Source: three-view drawing plus pictorial views. Frame: mm from the lowest corner of the part. Round coordinates to 2 decimals unless told otherwise and drop trailing zeros. Order: outer loops, then holes, each group sorted by start corner. A loop starts at its lowest first (then second) coordinate and runs counter-clockwise, first axis right, second up. Notation, with made-up numbers: (82.25, -31.5) -> (117.25, -31.5) arc R13 ccw to (117.25, -7.5) -> close; hole circle Ø6 at (8, -32). An arc over 180 degrees is marked (long way). Answer as CSV lines item,"result". Start each with the question number.
1) Line query: L1, parallel to Y at x = 105, z = 2.1; L2, parallel to X at y = 45, z = 2.2; L3, parallel to Y at x = 45, z = 1.8. Output: solid intervals per line, ascending.
2) Section query A-A, the plane y = 49.5. Output: boundary loops of the cut face in (x, z), and give its area (3 significant figures).
3) First-contact query: P1, Ø4, axis at x = 120, y = 60, coming from the +Z side. Flat tip, straight axial feed; report the tip coordinate or a pass-through.
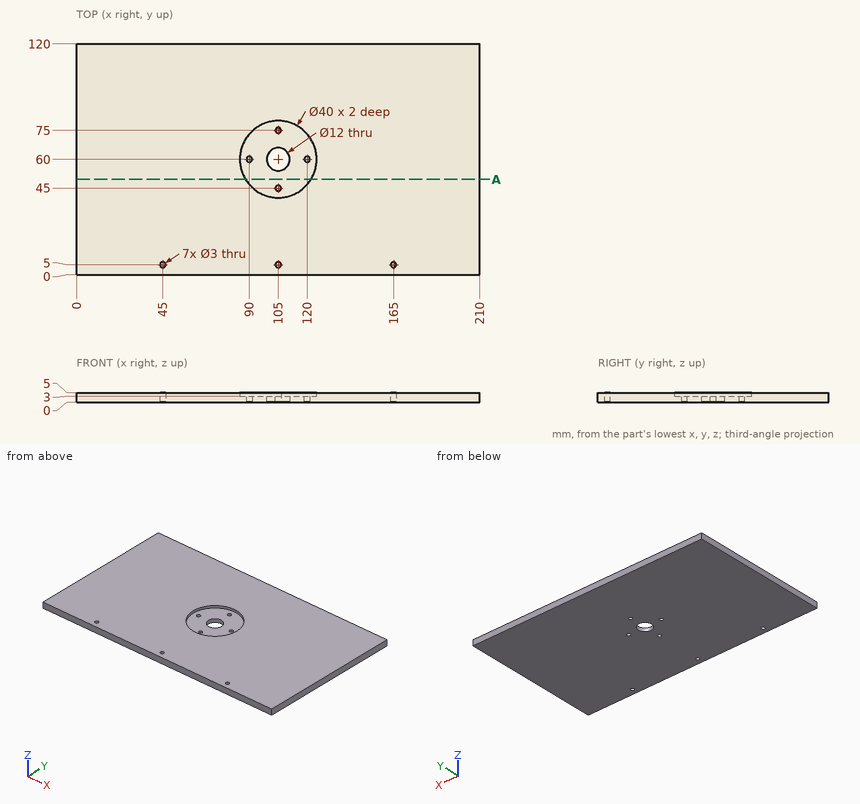
Findings:
1,L1,"y = 0 to 3.5, 6.5 to 43.5, 46.5 to 54, 66 to 73.5, 76.5 to 120"
1,L2,"x = 0 to 103.5, 106.5 to 210"
1,L3,"y = 0 to 3.5, 6.5 to 120"
2,outline,"(0, 0) -> (210, 0) -> (210, 5) -> (122.02, 5) -> (122.02, 3) -> (87.98, 3) -> (87.98, 5) -> (0, 5) -> close"
2,area,"982 mm^2"
3,P1,"stops at z = 3"
